Geometry: final body of the model. Coordinates: model frame, mm. Give positions to 0.01 mm unless a question says otherwise; leave off trailing zeros. Loops run counter-clockwise (first coordinate to the right, second up) from the corner with the lowest first, then second, coordinate; pieces in that order, holes last. Notation, with made-up numbers: (75.5, 81) - (107.5, 81) arc R25 cw to (107.5, 114) - close; hole circle Ø10 at (-10, 13.25). An arc over 180 degrees is marked (long way). Answer in a Markdown table with one row per item.
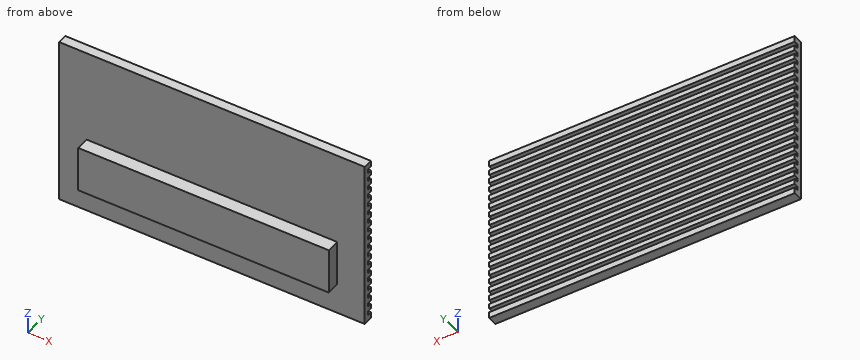
from build123d import *

# Parameters (mm, degrees)
BOSS_EXTRUDE1_DEPTH      = 2.1
BOSS_EXTRUDE1_DEPTH_BACK = 0.0001
SKETCH1_W                = 128
SKETCH1_H                = 71.5
SKETCH2_W                = 128
SKETCH2_H                = 2.6
BOSS_EXTRUDE2_DEPTH      = 1.8999
SKETCH3_W                = 128
SKETCH3_H                = 2.1
BOSS_EXTRUDE3_DEPTH      = 1.8999
LPATTERN1_COUNT          = 17
LPATTERN1_PITCH          = 3.803125
SKETCH6_W                = 105
SKETCH6_H                = 19.25
BOSS_EXTRUDE4_DEPTH      = 5.5


with BuildPart() as part:
    # Sketch1 → Boss-Extrude1 (new, two sides: drawn at the far end of the back side and taken through both)
    with BuildSketch(Plane(origin=(0, 0, 0), x_dir=(1, 0, 0), z_dir=(0, 1, 0)).offset(-BOSS_EXTRUDE1_DEPTH_BACK)):
        Rectangle(SKETCH1_W, SKETCH1_H)
    extrude(amount=BOSS_EXTRUDE1_DEPTH + BOSS_EXTRUDE1_DEPTH_BACK)

    # Sketch2 → Boss-Extrude2 (add)
    with BuildSketch(Plane(origin=(0, 2.1, 0), x_dir=(1, 0, 0), z_dir=(0, 1, 0))):
        with Locations((0, -34.45)):
            Rectangle(SKETCH2_W, SKETCH2_H)
        with Locations((0, 34.45)):
            Rectangle(SKETCH2_W, SKETCH2_H)
    extrude(amount=BOSS_EXTRUDE2_DEPTH)

    # Sketch3 → Boss-Extrude3 (add)
    with BuildSketch(Plane(origin=(0, 2.1, 0), x_dir=(1, 0, 0), z_dir=(0, 1, 0))):
        with Locations((0, -30.4)):
            Rectangle(SKETCH3_W, SKETCH3_H)
    boss_extrude3 = extrude(amount=BOSS_EXTRUDE3_DEPTH)

    # LPattern1: Boss-Extrude3 ×17
    with Locations(*[(0, 0, -i * LPATTERN1_PITCH) for i in range(1, LPATTERN1_COUNT)]):
        add(boss_extrude3)

    # Sketch6 → Boss-Extrude4 (add)
    with BuildSketch(Plane.XZ.offset(0.0001)):
        with Locations((0, -13.15)):
            Rectangle(SKETCH6_W, SKETCH6_H)
    extrude(amount=BOSS_EXTRUDE4_DEPTH)


solid = part.part
Q1. First-contact query: pin 1 (4 mm diameter, centred on x = 43, z = 6, fed in from -Y); pin 2 (0.5 mm diameter, centred on x = 17.5, z = 13, fed in from +Y). Flat tips, straight axial feed; report the tip coordinate or a pass-through.
Check values:
| item | result |
|---|---|
| pin 1 | y = 0 |
| pin 2 | y = 2.1 |
Q2. Cut plane A-A (y = -2.5). Output: boundary loops of the cut face in (x, z) (3 decimals), and give its area (3 significant figures).
Check values:
| item | result |
|---|---|
| outline | (-52.5, -22.775) - (52.5, -22.775) - (52.5, -3.525) - (-52.5, -3.525) - close |
| area | 2,020 mm² |
Q3. Material intervals for line 1 along Y through (x, z) = (-29, 27.5); line 2 along Z through (x, y) = (44, -1) (3 decimals); line 3 along Y through (x, z) = (-55.5, -13), sorted ascending.
Check values:
| item | result |
|---|---|
| line 1 | 0 to 4 |
| line 2 | -22.775 to -3.525 |
| line 3 | 0 to 2.1 |
